Part print with two shaded views. Sizes in mm from the minimum x, y, z corner. A direction names the side the tool comes from. Round coordinates to 2 decimals unless told otherwise and drop trailing zeros. Write each loop counter-clockwise with the first axis right and the second up, starting at its lowest first coordinate (ties: lowest second). Pieces come first, ordered by that corner, then holes. Notation, with made-up numbers: (-14, 88.5) - (31, 88.5) arc R25 cw to (31, 106.5) - close; hole circle Ø4 at (-38, -9). An arc over 180 degrees is marked (long way). Use one line per item in the form item = value. Start each with the question number.
Item 1: Band-saw the part on D-D, the plane x = 20. List the corners of the cut face in (y, z).
Item 2: Pull direction Z, two halves, no side cores. Call the marked faces 6, 7 and 8: +Z half, -Z half, draft (parallel to the pull), parting line (faces both ways), or undercut.
Item 3: Drill centre lines: L1, parallel to Z at x = 103.5, y = 1.5; L2, parallel to Z at x = 153, y = 6.5 (1 decimal); L3, parallel to Z at x = 20, y = 13.5. Where is each one in solid material? Low to high.
Item 4: Pin check, flat tips, straight feed: pin 1 (6 mm diameter, centred on x = 98.5, y = 4.5, fed in from +Z); pin 2 (8 mm diameter, centred on y = 16, z = 35.5, fed in from -X); pin 3 (6 mm diameter, centred on y = 15, z = 21.5, fed in from -X); pin 4 (8 mm diameter, centred on x = 50.5, y = 4.5, fed in from -Z). Stop position of each tip, or through.
Item 5: Band-saw the part on A-A, the plane x = 81.5. List the corners of the cut face in (y, z), and give its area (3 significant figures).
Item 6: Band-saw the part on C-C, the plane x = 149.5. List the corners of the cut face in (y, z).
Item 7: Tool access for the marked faces 1, 2, 3, 4 and 5: list every direction of +Z, -Z, +X, -X, +Y, -Y with a clear straight run to the whole face (end or side of a thin tool).
Item 8: Band-saw the part on B-B, the plane y = 12.5. List the corners of the cut face in (x, z).
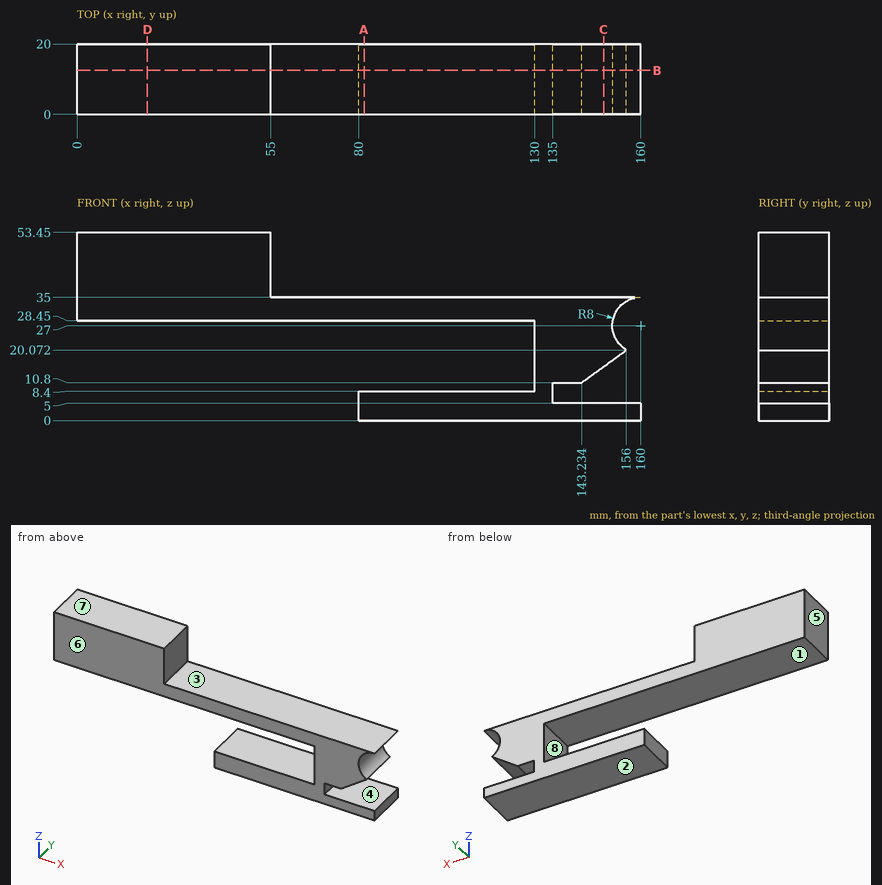
Determined:
q1.outline = (0, 28.45) - (20, 28.45) - (20, 53.45) - (0, 53.45) - close
q2.face_6 = draft
q2.face_7 = +Z half
q2.face_8 = undercut
q3.L1 = 0 to 8.4, 28.45 to 35
q3.L2 = 0 to 5, 17.9 to 23.1, 30.9 to 35
q3.L3 = 28.45 to 53.45
q4.pin_1 = 35
q4.pin_2 = 0
q4.pin_3 = 130
q4.pin_4 = 28.45
q5.outline = (0, 0) - (20, 0) - (20, 8.4) - (0, 8.4) - close; (0, 28.45) - (20, 28.45) - (20, 35) - (0, 35) - close
q5.area = 299 mm²
q6.outline = (0, 0) - (20, 0) - (20, 5) - (0, 5) - close; (0, 15.35) - (20, 15.35) - (20, 35) - (0, 35) - close
q7.face_1 = -X, +Y, -Y
q7.face_2 = -Z, +X, -X, +Y, -Y
q7.face_3 = +Z, +X, +Y, -Y
q7.face_4 = +X, +Y, -Y
q7.face_5 = +Z, -Z, -X, +Y, -Y
q8.outline = (0, 28.45) - (130, 28.45) - (130, 8.4) - (80, 8.4) - (80, 0) - (160, 0) - (160, 5) - (135, 5) - (135, 10.8) - (143.23, 10.8) - (156, 20.07) arc R8 cw to (160, 35) - (55, 35) - (55, 53.45) - (0, 53.45) - close
